Build history of the part. All positions in model axes, mm. Face numbers are marked on the shaded views. Round coordinates to 2 decimals unless told otherwise and drop trailing zeros. Write each loop counter-clockwise with the first axis right and the second up, starting at its lowest first coordinate (ties: lowest second). Pieces come first, ordered by that corner, then holes.
1) Saw through at A-A (z = 40). Write the cut outline in (x, y).
2) Flat gauge pins, fed straight in: pin 1 (6 mm diameter, centred on x = 12, z = 33, fed in from -Y); pin 2 (5.5 mm diameter, centred on x = -15.5, y = -46.5, fed in from -Z). Where does each tip first touch, or does it go through?
3) Saw through at B-B (y = -3). Write the cut outline in (x, z), plus the area to 3 significant figures.
4) Saw through at D-D (y = -25). Write the cut outline in (x, z), plus the area to 3 significant figures.
5) Saw through at C-C (x = -47.5). Write the cut outline in (y, z), plus the area to 3 significant figures.
6) Pull direction X, two halves, no side cores. Call the marked faces 1 and 2: +X half, -X half, draft (parallel to the pull), parting line (faces both ways), or undercut.
7) Wall check: probe 1 along Z at (x, y) = (-53.5, -20.5). Give the ranges that are in metal, low to high.
from build123d import *

# Parameters (mm, degrees)
F0_W     = 100.2733111382
F0_H     = 50.1366546378
F1_DEPTH = 50
F2_W     = 90.2733111382
F2_H     = 8.7347067715
F3_DEPTH = 50.001
F5_W     = 40.5144635588
F5_H     = 41.020902805
F6_DEPTH = 100.2743111382
F7_W     = 89.8914821446
F7_H     = 32.1583626792
F8_DEPTH = 50.001


with BuildPart() as f1:
    # F0 (on Front) → F1 (new body)
    with BuildSketch(Plane.XZ):
        with Locations((-15.6993567944, 31.3960765488)):
            Rectangle(F0_W, F0_H)
    extrude(amount=F1_DEPTH)

    # F2 (on face) → F3 (cut, through all)
    with BuildSketch(Plane.XZ.offset(50)):
        with Locations((-15.6993567944, 47.097050482)):
            Rectangle(F2_W, F2_H)
    extrude(amount=-F3_DEPTH, mode=Mode.SUBTRACT)

    # F5 (on face) → F6 (cut, through all)
    with BuildSketch(Plane(origin=(-65.8360123634, 0, 0), x_dir=(0, -1, 0), z_dir=(-1, 0, 0))):
        with Locations((24.5618959889, 29.3703549542)):
            Rectangle(F5_W, F5_H)
    extrude(amount=-F6_DEPTH, mode=Mode.SUBTRACT)

    # F7 (on face) → F8 (cut, through all)
    with BuildSketch(Plane.XZ.offset(50)):
        with Locations((-16.0791818053, 22.4069305696)):
            Rectangle(F7_W, F7_H)
    extrude(amount=-F8_DEPTH, mode=Mode.SUBTRACT)


solid = f1.part
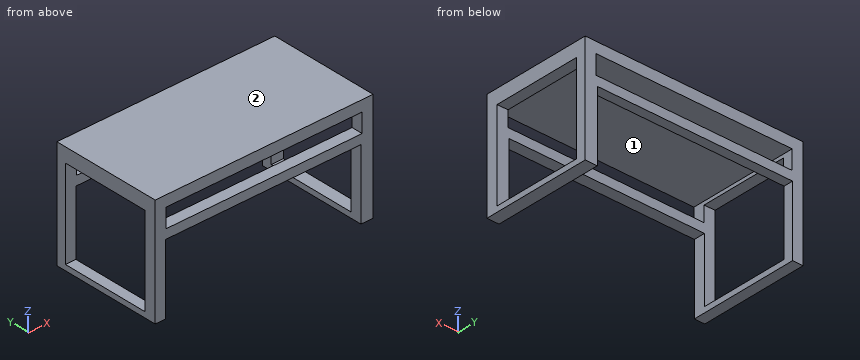
Evaluation:
1. outline: (-65.84, -50) - (34.44, -50) - (34.44, -44.82) - (-65.84, -44.82) - close; (-65.84, -4.3) - (34.44, -4.3) - (34.44, 0) - (-65.84, 0) - close
2. pin 1: passes through
2. pin 2: stops at z = 38.49
3. outline: (-65.84, 6.33) - (-61.02, 6.33) - (-61.02, 38.49) - (28.87, 38.49) - (28.87, 6.33) - (34.44, 6.33) - (34.44, 56.46) - (-65.84, 56.46) - close; hole (-60.84, 42.73) - (29.44, 42.73) - (29.44, 51.46) - (-60.84, 51.46) - close
3. area: 1,350 mm2
4. outline: (-65.84, 6.33) - (-61.02, 6.33) - (-61.02, 8.86) - (-65.84, 8.86) - close; (-65.84, 49.88) - (-60.84, 49.88) - (-60.84, 51.46) - (29.44, 51.46) - (29.44, 49.88) - (34.44, 49.88) - (34.44, 56.46) - (-65.84, 56.46) - close; (28.87, 6.33) - (34.44, 6.33) - (34.44, 8.86) - (28.87, 8.86) - close
4. area: 543 mm2
5. outline: (-50, 38.49) - (-44.82, 38.49) - (-44.82, 42.73) - (-50, 42.73) - close; (-50, 51.46) - (0, 51.46) - (0, 56.46) - (-50, 56.46) - close; (-4.3, 38.49) - (0, 38.49) - (0, 42.73) - (-4.3, 42.73) - close
5. area: 290 mm2
6. face 1: undercut
6. face 2: draft
7. probe 1: z = 51.46 to 56.46
